```python
from build123d import *

# Parameters (mm, degrees)
SKETCH1_R        = 41.275
SKETCH1_R_2      = 38.1
SKETCH1_R_3      = 2.54
SKETCH1_R_4      = 9.525
BASE_DEPTH       = 2.54
SKETCH2_R        = 41.275
SKETCH2_R_2      = 38.1
FRONT_WALL_DEPTH = 3.175


with BuildPart() as part:
    # Sketch1 → base (new body)
    with BuildSketch(Plane(origin=(0, 0, 0), x_dir=(1, 0, 0), z_dir=(0, 1, 0))):
        with Locations(Location((0, 0, 0), (0, 0, 270))):
            Circle(SKETCH1_R)
        Circle(SKETCH1_R_2, mode=Mode.SUBTRACT)
        Circle(SKETCH1_R_2)
        with Locations(Location((-25.4, 0, 0), (0, 0, 270))):
            Circle(SKETCH1_R_3, mode=Mode.SUBTRACT)
        with Locations(Location((0, -25.4, 0), (0, 0, 270))):
            Circle(SKETCH1_R_3, mode=Mode.SUBTRACT)
        with Locations(Location((25.4, 0, 0), (0, 0, 270))):
            Circle(SKETCH1_R_3, mode=Mode.SUBTRACT)
        with Locations(Location((0, 25.4, 0), (0, 0, 270))):
            Circle(SKETCH1_R_3, mode=Mode.SUBTRACT)
        with Locations(Location((0, 0, 0), (0, 0, 270))):
            Circle(SKETCH1_R_4, mode=Mode.SUBTRACT)
    extrude(amount=BASE_DEPTH)

    # Sketch2 → front wall (add)
    with BuildSketch(Plane(origin=(0, 2.54, 0), x_dir=(1, 0, 0), z_dir=(0, 1, 0))):
        with Locations(Location((0, 0, 0), (0, 0, 270))):
            Circle(SKETCH2_R)
        with Locations(Location((0, 0, 0), (0, 0, 270))):
            Circle(SKETCH2_R_2, mode=Mode.SUBTRACT)
    extrude(amount=FRONT_WALL_DEPTH)


solid = part.part
```
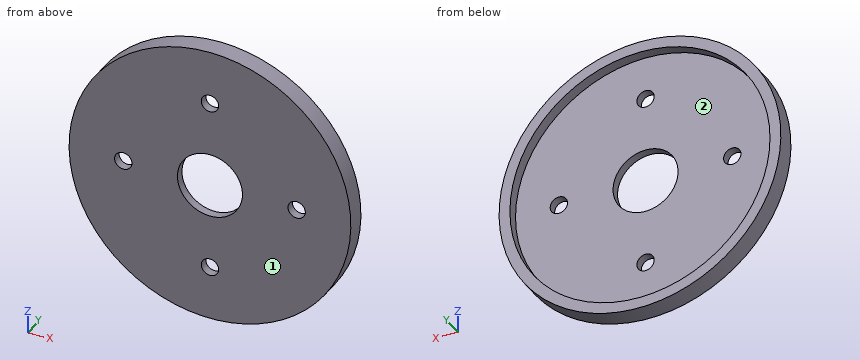
Read the model definition and answer for the solid it produces. Units are mm, in the model's axes. Face numbers are marked on the shaded views. Coordinates: 2 decimals unless noted, no trailing zeros. Order: outer loops, then holes, each group sorted by start corner. A loop starts at its lowest first (then second) coordinate and runs counter-clockwise, first axis right, second up. Notation, with made-up numbers: (35, 80) - (73, 80) arc R17 cw to (73, 97) - close; hole circle Ø8 at (-31, -8). An arc over 180 degrees is marked (long way). Answer as a JSON object with one key per item and string values. Group by question number.
Item 1: Flat-ended cylindrical pins translate along their axes: P1, Ø8, axis at x = 0, z = 25.4, coming from the +Y side; P2, Ø1, axis at y = 2, z = -13, coming from the +X side; P3, Ø4.5, axis at x = -25.4, z = 0, coming from the -Y side; P4, Ø2, axis at y = 2, z = 9, coming from the +X side. Find the tip coordinate at first contact, or state that the pin passes through.
Item 2: Consider probe 1 along X at (y, z) = (1.6, 0) (3 decimals); probe 2 along Z at (x, y) = (1, 5.35); probe 3 along Y at (x, z) = (37, 1.5). Determine where each line is inside the solid, lowest interval first. Write a range as from..to.
Item 3: The mould has two halves that part along Z. Classify the marked faces 1 and 2: +Z half, -Z half, draft (parallel to the pull), parting line (faces both ways), or undercut.
Item 4: Section C-C (y = 4.35) is taken. Give the vertices of the cut face in (x, z) (3 decimals).
Item 5: Section A-A (x = 0) is taken. Give the vertices of the cut face in (y, z) (3 decimals).
Item 6: Section D-D (x = 25.4) is taken. Give the vertices of the cut face in (y, z) (3 decimals).
Item 7: Section B-B (z = -8) is taken. Give the vertices of the cut face in (x, y) (3 decimals), plus the area to 3 significant figures.
Results are:
{
 "1": {"P1": "stops at y = 2.54", "P2": "stops at x = 39.34", "P3": "passes through", "P4": "stops at x = 40.49"},
 "2": {"probe 1": "x = -41.275..-27.94, -22.86..-9.525, 9.525..22.86, 27.94..41.275", "probe 2": "z = -41.26..-38.09, 38.09..41.26", "probe 3": "y = 0..2.54"},
 "3": {"face 1": "draft", "face 2": "undercut"},
 "4": {"outline": "circle Ø82.55 at (0, 0); hole circle Ø76.2 at (0, 0)"},
 "5": {"outline": "(0, -41.275) - (5.715, -41.275) - (5.715, -38.1) - (2.54, -38.1) - (2.54, -27.94) - (0, -27.94) - close; (0, -22.86) - (2.54, -22.86) - (2.54, -9.525) - (0, -9.525) - close; (0, 9.525) - (2.54, 9.525) - (2.54, 22.86) - (0, 22.86) - close; (0, 27.94) - (2.54, 27.94) - (2.54, 38.1) - (5.715, 38.1) - (5.715, 41.275) - (0, 41.275) - close"},
 "6": {"outline": "(0, -32.534) - (5.715, -32.534) - (5.715, -28.398) - (2.54, -28.398) - (2.54, -2.54) - (0, -2.54) - close; (0, 2.54) - (2.54, 2.54) - (2.54, 28.398) - (5.715, 28.398) - (5.715, 32.534) - (0, 32.534) - close"},
 "7": {"outline": "(-40.492, 0) - (-5.17, 0) - (-5.17, 2.54) - (-37.251, 2.54) - (-37.251, 5.715) - (-40.492, 5.715) - close; (5.17, 0) - (40.492, 0) - (40.492, 5.715) - (37.251, 5.715) - (37.251, 2.54) - (5.17, 2.54) - close", "area": "200 mm^2"}
}
